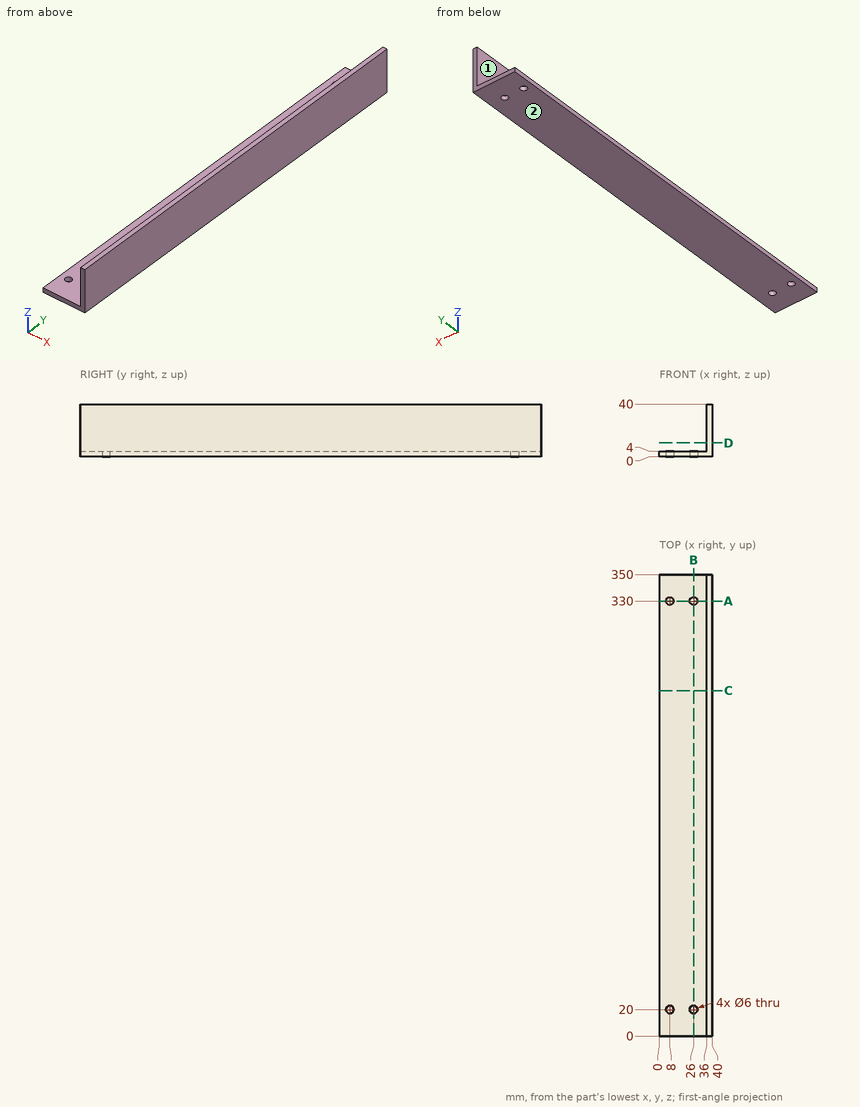
Input: dimensioned drawing with shaded views. Units: mm. Origin: part minimum x, y, z. A direction names the side the tool comes from. Give positions to 0.01 mm unless a question says otherwise; leave off trailing zeros. Write each loop counter-clockwise with the first axis right and the second up, starting at its lowest first coordinate (ties: lowest second). Pieces come first, ordered by that corner, then holes. Notation, with made-up numbers: (-19.75, 14.5) - (-1.75, 14.5) arc R7 ccw to (-1.75, 26.5) - close; hole circle Ø3 at (20.5, 60). An arc over 180 degrees is marked (long way). One line per item, written item: value. Start each with the question number.
Q1. Section query C-C, the plane y = 262. Return the cut outline in (x, z).
Q2. Material intervals for probe 1 along Y at (x, z) = (26, 2); probe 2 along X at (y, z) = (330, 2); probe 3 along Z at (x, y) = (27.5, 92), sorted ascending. Write a range as from..to.
Q3. Set-up query: the marked faces 1 and 2. Return all of +Z, -Z, +X, -X, +Y, -Y with unobstructed straight access to the full face (end or side cutting, diameter ignored); none if empty.
Q4. Section query D-D, the plane z = 10.5. Return the cut outline in (x, y).
Q5. Section query B-B, the plane x = 26. Return the cut outline in (y, z).
Q6. First-contact query: pin 1 Ø7 at (x, y) = (26, 330) entering from -Z; pin 2 Ø11 at (x, y) = (24, 234) entering from +Z; pin 3 Ø18 at (y, z) = (166.5, 20.5) entering from -X. Flat tips, straight axial feed; report the tip coordinate or a pass-through.
Q7. Section query A-A, the plane y = 330. Return the cut outline in (x, z).
Answer:
1. outline: (0, 0) - (40, 0) - (40, 40) - (36, 40) - (36, 4) - (0, 4) - close
2. probe 1: y = 0..17, 23..327, 333..350
2. probe 2: x = 0..5, 11..23, 29..40
2. probe 3: z = 0..4
3. face 1: +Z, -X, +Y, -Y
3. face 2: -Z, +X, -X, +Y, -Y
4. outline: (36, 0) - (40, 0) - (40, 350) - (36, 350) - close
5. outline: (0, 0) - (17, 0) - (17, 4) - (0, 4) - close; (23, 0) - (327, 0) - (327, 4) - (23, 4) - close; (333, 0) - (350, 0) - (350, 4) - (333, 4) - close
6. pin 1: stops at z = 0
6. pin 2: stops at z = 4
6. pin 3: stops at x = 36
7. outline: (0, 0) - (5, 0) - (5, 4) - (0, 4) - close; (11, 0) - (23, 0) - (23, 4) - (11, 4) - close; (29, 0) - (40, 0) - (40, 40) - (36, 40) - (36, 4) - (29, 4) - close
